Work out the finished part from the listing and answer in its coordinate system (mm). Face numbers are marked on the shaded views. A direction names the side the tool comes from. Round coordinates to 2 decimals unless told otherwise and drop trailing zeros. Write each loop counter-clockwise with the first axis right and the second up, starting at its lowest first coordinate (ties: lowest second). Pieces come first, ordered by that corner, then holes.
1. A tool of negligible diameter and unlimited length cuts with its end or side. For the marked faces 1, 2, 3 and 4, from which of +Z, -Z, +X, -X, +Y, -Y can it reach the whole face along a straight path? Write none if from no direction.
2. Find section D-D (z = -16). Write down the section's boundary in (x, y), and give its area (3 significant figures).
3. Determine the mould class of the marked faces 5, 6, 7 and 8 for opening direction Z: pulls with the +Z half, pulls with the -Z half, needs draft (parallel to the pull), parting line crosses it, or undercut.
4. Find section A-A (z = 19.5). Write down the section's boundary in (x, y).
5. Straight lines are drawn through the part: probe 1 along X at (y, z) = (1, -13); probe 2 along Z at (x, y) = (8.5, -25.5); probe 3 along Z at (x, y) = (-9.5, 1). For each, find the intervals that lie inside material, in ascending order.
6. Flat-ended cylindrical pins translate along their axes: pin 1 Ø9 at (x, y) = (2, -20) entering from -Z; pin 2 Ø11 at (y, z) = (-20.5, -9.5) entering from +X; pin 3 Ø20 at (x, z) = (2.5, -2) entering from -Y; pin 4 Ø9 at (x, y) = (-2.5, -8) entering from +Z. Find the tip coordinate at first contact, or state that the pin passes through.
7. Find section C-C (y = -19). Write down the section's boundary in (x, z).
8. Find section B-B (x = -1). Write down the section's boundary in (y, z), and give its area (3 significant figures).
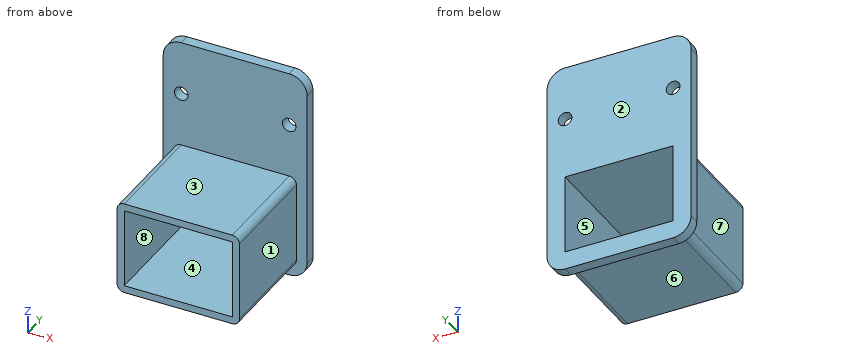
Autodesk Inventor part; units mm, degrees
ref_plane "YZ Plane" through (0, 0, 0) normal (1, 0, 0) x (0, 1, 0)
ref_plane "XZ Plane" through (0, 0, 0) normal (0, 1, 0) x (-1, 0, 0)
ref_plane "XY Plane" through (0, 0, 0) normal (0, 0, 1) x (1, 0, 0)
sketch "Sketch1" plane through (0, 0, 0) normal (0, 1, 0) x (-1, 0, 0)
  line L0 (-20, 24.5) -> (20, 24.5)
  line L1 (20, 24.5) -> (20, -24.5)
  line L2 (20, -24.5) -> (-20, -24.5)
  line L3 (-20, -24.5) -> (-20, 24.5)
  line L4 (-20, 24.5) -> (20, -24.5) construction
  line L5 (20, 24.5) -> (-20, -24.5) construction
  circle A0 centre (15, 19.5) radius 1.9
  circle A1 centre (-15, 19.5) radius 1.9
  line L6 (15, 2.5) -> (-15, 2.5)
  line L7 (-15, 2.5) -> (-15, -19.5)
  line L8 (-15, -19.5) -> (15, -19.5)
  line L9 (15, -19.5) -> (15, 2.5)
  line L10 (15, 2.5) -> (-15, -19.5) construction
  line L11 (-15, 2.5) -> (15, -19.5) construction
  point P0 (0, 0)
  point P1 (15, 17.5)
  point P2 (-15, 17.5)
  point P3 (0, -8.5)
  point P4 (0, -8.5)
  point P5 (0, 0)
  dimension "d0" = 30
  dimension "d1" = 3.8
  dimension "d4" = 5
  dimension "d5" = 15
  dimension "d6" = 22
  dimension "d7" = 30
  dimension "d9" = 49
  dimension "d12" = 40
  dimension "d21" = 22
extrude "Extrusion1" add sketch "Sketch1" along normal blind 3
sketch "Sketch2" plane through (0, 0, 0) normal (0, -1, 0) x (1, 0, 0)
  point P0 (0, 0)
sketch "Sketch3" plane through (0, 0, 0) normal (0, -1, 0) x (1, 0, 0)
  line L0 (17, -21.5) -> (-17, -21.5)
  line L1 (-17, -21.5) -> (-17, 4.5)
  line L2 (-17, 4.5) -> (17, 4.5)
  line L3 (17, 4.5) -> (17, -21.5)
  line L4 (17, -21.5) -> (-17, 4.5) construction
  line L5 (-17, -21.5) -> (17, 4.5) construction
  line L6 (-15, -19.5) -> (-15, 2.5)
  line L7 (15, 2.5) -> (15, -19.5)
  line L8 (15, -19.5) -> (-15, -19.5)
  line L9 (-15, 2.5) -> (15, 2.5)
  line L10 (15, 2.5) -> (-15, 2.5)
  line L11 (15, -19.5) -> (-15, -19.5)
  line L12 (-15, -19.5) -> (-15, 2.5)
  line L13 (-15, 2.5) -> (15, 2.5)
  line L14 (15, 2.5) -> (15, -19.5)
  line L15 (15, -19.5) -> (-15, 2.5) construction
  line L16 (-15, -19.5) -> (15, 2.5) construction
  point P0 (0, 0)
  point P1 (0, -8.5)
  point P2 (0, -8.5)
  dimension "d13" = 2
  dimension "d14" = 2
  dimension "d15" = 2
  dimension "d16" = 2
extrude "Extrusion2" add sketch "Sketch3" along normal blind 30
fillet "Fillet1" radius 5 4 edges at (-20, 1.5, -24.5) (-20, 1.5, 24.5) (20, 1.5, 24.5) (20, 1.5, -24.5)
fillet "Fillet2" radius 2 4 edges at (-17, -15, -21.5) (17, -15, 4.5) (-17, -15, 4.5) (17, -15, -21.5)
sketch "Sketch4" plane through (0, 3, 0) normal (0, 1, 0) x (1, 0, 0)
  line L0 (-15, -24.5) -> (15, -24.5)
  arc A0 (15, -24.5) -> (20, -19.5) centre (15, -19.5) ccw
  arc A1 (-20, -19.5) -> (-15, -24.5) centre (-15, -19.5) ccw
  line L1 (20, -19.5) -> (-20, -19.5)
  line L2 (-20, -19.5) -> (-20, -34.5)
  line L3 (-20, -34.5) -> (20, -34.5)
  line L4 (20, -34.5) -> (20, -19.5)
  point P0 (0, 0)
  dimension "d22" = 15
extrude "Extrusion3" add sketch "Sketch4" against normal up to surface (3 mm away) contours L0 A0 L4 L3 L2 A1
fillet "Fillet3" radius 5 2 edges at (20, 1.5, 34.5) (-20, 1.5, 34.5)
properties part number "ButtonBox"
Worked answers:
1. face 1: +Z, -Z, +X, -Y
1. face 2: +Z, -Z, +X, -X, +Y
1. face 3: +Z, +X, -X, -Y
1. face 4: +Y, -Y
2. outline: (-20, 0) - (-17, 0) - (-17, -30) - (-15, -30) - (-15, 3) - (-20, 3) - close; (15, -30) - (17, -30) - (17, 0) - (20, 0) - (20, 3) - (15, 3) - close
2. area: 150 mm2
3. face 5: undercut
3. face 6: pulls with the -Z half
3. face 7: needs draft
3. face 8: undercut
4. outline: (-20, 0) - (-16.9, 0) - (-16.9, 3) - (-20, 3) - close; (-13.1, 0) - (13.1, 0) - (13.1, 3) - (-13.1, 3) - close; (16.9, 0) - (20, 0) - (20, 3) - (16.9, 3) - close
5. probe 1: x = -20 to -15, 15 to 20
5. probe 2: z = -21.5 to -19.5, 2.5 to 4.5
5. probe 3: z = -24.5 to -19.5, 2.5 to 34.5
6. pin 1: stops at z = -21.5
6. pin 2: stops at x = 17
6. pin 3: stops at y = -30
6. pin 4: stops at z = 4.5
7. outline: (-17, -19.5) arc R2 ccw to (-15, -21.5) - (15, -21.5) arc R2 ccw to (17, -19.5) - (17, 2.5) arc R2 ccw to (15, 4.5) - (-15, 4.5) arc R2 ccw to (-17, 2.5) - close; hole (-15, -19.5) - (15, -19.5) - (15, 2.5) - (-15, 2.5) - close
8. outline: (-30, -21.5) - (0, -21.5) - (0, -24.5) - (3, -24.5) - (3, -19.5) - (-30, -19.5) - close; (-30, 2.5) - (3, 2.5) - (3, 34.5) - (0, 34.5) - (0, 4.5) - (-30, 4.5) - close
8. area: 231 mm2
